Can you work these out from the model? Positions are in its coordinate system, mm. Coordinates: 2 decimals unless noted, no trailing zeros. Order: outer loops, then holes, each group sorted by start corner. A loop starts at its lowest first (then second) coordinate and runs counter-clockwise, first axis right, second up. Notation, with made-up numbers: M 75.25,30.25 L 85.25,30.25 A38 cw 85.25,69.25 Z; hole C 35,3.25 d2. An arc over 180 degrees is marked long. Answer as a JSON object with one key per item and string values.
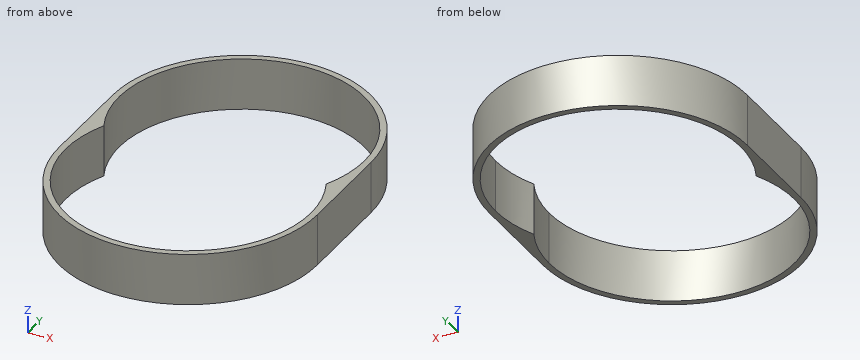
from build123d import *

# Parameters (mm, degrees)
F2_DEPTH = 20
F3_DEPTH = 20
F4_DEPTH = 20


with BuildPart() as f2:
    # F1 (on Top) → F2 (new body)
    with BuildSketch(Plane.XY):
        with BuildLine():
            ThreePointArc((-45.8257569496, -20), (0, -50), (45.8257569496, -20))
            ThreePointArc((45.8257569496, -20), (0, 10), (-45.8257569496, -20))
        make_face()
    extrude(amount=F2_DEPTH)

    # F1 (on Top) → F3 (join)
    with BuildSketch(Plane.XY):
        with BuildLine():
            ThreePointArc((45.8257569496, -20), (48.9453156465, -10.2154821845), (50, 0))
            ThreePointArc((50, 0), (0, 50), (-50, 0))
            ThreePointArc((-50, 0), (-48.9453156465, -10.2154821845), (-45.8257569496, -20))
            ThreePointArc((-45.8257569496, -20), (0, 10), (45.8257569496, -20))
        make_face()
        with BuildLine():
            Line((50, -40), (50, 0))
            ThreePointArc((50, 0), (48.9453156465, -10.2154821845), (45.8257569496, -20))
            ThreePointArc((45.8257569496, -20), (48.9453156465, -29.7845178155), (50, -40))
        make_face()
        with BuildLine():
            ThreePointArc((-45.8257569496, -20), (-48.9453156465, -10.2154821845), (-50, 0))
            Line((-50, 0), (-50, -40))
            ThreePointArc((-50, -40), (-48.9453156465, -29.7845178155), (-45.8257569496, -20))
        make_face()
        with BuildLine():
            ThreePointArc((50, -40), (48.9453156465, -29.7845178155), (45.8257569496, -20))
            ThreePointArc((45.8257569496, -20), (0, -50), (-45.8257569496, -20))
            ThreePointArc((-45.8257569496, -20), (-48.9453156465, -29.7845178155), (-50, -40))
            ThreePointArc((-50, -40), (0, -90), (50, -40))
        make_face()
    extrude(amount=F3_DEPTH)

    # F0 (on Top) → F4 (cut)
    with BuildSketch(Plane.XY):
        with BuildLine():
            ThreePointArc((43.084219849, -20), (46.3829195008, -10.2408387638), (47.5, 0))
            ThreePointArc((47.5, 0), (-10.2408387638, 46.3829195008), (-43.084219849, -20))
            ThreePointArc((-43.084219849, -20), (0, 7.5), (43.084219849, -20))
        make_face()
        with BuildLine():
            ThreePointArc((43.084219849, -20), (0, 7.5), (-43.084219849, -20))
            ThreePointArc((-43.084219849, -20), (0, -47.5), (43.084219849, -20))
        make_face()
        with BuildLine():
            ThreePointArc((43.084219849, -20), (0, -47.5), (-43.084219849, -20))
            ThreePointArc((-43.084219849, -20), (-10.2408387638, -86.3829195008), (47.5, -40))
            ThreePointArc((47.5, -40), (46.3829195008, -29.7591612362), (43.084219849, -20))
        make_face()
    extrude(amount=F4_DEPTH, mode=Mode.SUBTRACT)


solid = f2.part
Item 1: I'm going to push flat-ended pins straight in: pin 1 (10 mm diameter, centred on x = 28.5, z = 10.5, fed in from -Y); pin 2 (10 mm diameter, centred on x = 18, z = 6.5, fed in from -Y); pin 3 (12 mm diameter, centred on x = 30.5, z = 4.5, fed in from +Y). Where does each tip first touch, or does it pass through?
Answers follow:
{"pin 1": "stops at y = -84.13", "pin 2": "stops at y = -88.28", "pin 3": "stops at y = 43.59"}
Item 2: Please list where these lines run through material, in increasing order: line 1 (Y direction, x = -29.5, z = 11.5); line 2 (X direction, y = -40, z = 4.75); line 3 (Y direction, x = -13.5, z = 17.25).
Answers follow:
{"line 1": "y = -80.37 to -77.23, 37.23 to 40.37", "line 2": "x = -50 to -47.5, 47.5 to 50", "line 3": "y = -88.14 to -85.54, 45.54 to 48.14"}
Item 3: I want a section at B-B, the plane y = -24. Write out the boundary of the cut face in (x, z).
Answers follow:
{"outline": "M -50,0 L -44.72,0 L -44.72,20 L -50,20 Z; M 44.72,0 L 50,0 L 50,20 L 44.72,20 Z"}
Item 4: I want a section at C-C, the plane z = 13. Write out the boundary of the cut face in (x, y).
Answers follow:
{"outline": "M -50,-40 A50 ccw 50,-40 L 50,0 A50 ccw -50,0 Z; hole M -43.08,-20 A47.5 ccw long 43.08,-20 A47.5 ccw long Z"}
Item 5: I want a section at A-A, the plane x = -33. Write out the boundary of the cut face in (y, z), plus the area to 3 significant figures.
Answers follow:
{"outline": "M -77.56,0 L -74.17,0 L -74.17,20 L -77.56,20 Z; M 34.17,0 L 37.56,0 L 37.56,20 L 34.17,20 Z", "area": "136 mm^2"}
